```python
from build123d import *

# Parameters (mm, degrees)
F0_W      = 25
F0_H      = 15
F1_DEPTH  = 6
F3_DEPTH  = 10
F5_D      = 5
F6_W      = 10
F6_H      = 15
F7_DEPTH  = 16
F8_DEPTH  = 25.4
F9_DEPTH  = 10
F10_R     = 1.75
F11_DEPTH = 10


with BuildPart() as f1:
    # F0 (on Top) → F1 (new body)
    with BuildSketch(Plane.XY):
        with BuildLine():
            ThreePointArc((-22.1608236432, 15), (-34.6608236432, 27.5), (-47.1608236432, 15))
            Line((-47.1608236432, 15), (-22.1608236432, 15))
        make_face()
        with Locations((-34.6608236432, 7.5)):
            Rectangle(F0_W, F0_H)
        with BuildLine():
            Line((-22.1608236432, 0), (-47.1608236432, 0))
            ThreePointArc((-47.1608236432, 0), (-34.6608236432, -12.5), (-22.1608236432, 0))
        make_face()
    extrude(amount=F1_DEPTH)

    # F2 (on Top) → F3 (join)
    with BuildSketch(Plane.XY):
        with BuildLine():
            Line((-17.1608236432, 0), (-17.1608236432, 15))
            ThreePointArc((-17.1608236432, 15), (-34.6608236432, 32.5), (-52.1608236432, 15))
            Line((-52.1608236432, 15), (-52.1608236432, 0))
            ThreePointArc((-52.1608236432, 0), (-34.6608236432, -17.5), (-17.1608236432, 0))
        make_face()
    extrude(amount=-F3_DEPTH)

    # F5 (through all)
    with Locations(Plane(origin=(-52.1608236432, 0, 0), x_dir=(0, -1, 0), z_dir=(-1, 0, 0))):
        with Locations((-7.5, -5)):
            Hole(F5_D / 2)

    # F6 (on face) → F7 (cut, through all)
    with BuildSketch(Plane(origin=(0, 0, -10), x_dir=(1, 0, 0), z_dir=(0, 0, -1))):
        Polygon((-39.6608236432, 1.5), (-39.6608236432, 0), (-29.6608236432, 0), (-29.6608236432, 1.5), (-34.6608236432, 1.5), align=None)
        with Locations((-34.6608236432, -7.5)):
            Rectangle(F6_W, F6_H)
        Polygon((-29.6608236432, -15), (-39.6608236432, -15), (-39.6608236432, -16.5), (-34.6608236432, -16.5), (-29.6608236432, -16.5), align=None)
    extrude(amount=-F7_DEPTH, mode=Mode.SUBTRACT)

    # F6 (on face) → F8 (cut)
    with BuildSketch(Plane(origin=(0, 0, -10), x_dir=(1, 0, 0), z_dir=(0, 0, -1))):
        with BuildLine():
            ThreePointArc((-30.6608236432, -22.5), (-31.8323965185, -19.6715728753), (-34.6608236432, -18.5))
            ThreePointArc((-34.6608236432, -18.5), (-37.489250768, -25.3284271247), (-30.6608236432, -22.5))
        make_face()
        with BuildLine():
            ThreePointArc((-30.6608236432, 7.5), (-37.489250768, 10.3284271247), (-34.6608236432, 3.5))
            ThreePointArc((-34.6608236432, 3.5), (-31.8323965185, 4.6715728753), (-30.6608236432, 7.5))
        make_face()
    extrude(amount=-F8_DEPTH, mode=Mode.SUBTRACT)

    # F6 (on face) → F9 (join)
    with BuildSketch(Plane(origin=(0, 0, -10), x_dir=(1, 0, 0), z_dir=(0, 0, -1))):
        with BuildLine():
            ThreePointArc((-30.6608236432, -22.5), (-31.8323965185, -19.6715728753), (-34.6608236432, -18.5))
            ThreePointArc((-34.6608236432, -18.5), (-37.489250768, -25.3284271247), (-30.6608236432, -22.5))
        make_face()
        with BuildLine():
            ThreePointArc((-30.6608236432, 7.5), (-37.489250768, 10.3284271247), (-34.6608236432, 3.5))
            ThreePointArc((-34.6608236432, 3.5), (-31.8323965185, 4.6715728753), (-30.6608236432, 7.5))
        make_face()
    extrude(amount=-F9_DEPTH)

    # F10 (on face) → F11 (cut)
    with BuildSketch(Plane.XY):
        with Locations((-34.6608236432, 30)):
            Circle(F10_R)
        with Locations((-34.6608236432, -15)):
            Circle(F10_R)
    extrude(amount=-F11_DEPTH, mode=Mode.SUBTRACT)


solid = f1.part
```
Could you check a few things on this model? Use its own coordinates, in mm. A direction names the side the tool comes from. Round coordinates to 2 decimals unless told otherwise and drop trailing zeros. Write each loop counter-clockwise with the first axis right and the second up, starting at its lowest first coordinate (ties: lowest second). Pieces come first, ordered by that corner, then holes. Notation, with made-up numbers: M 7,35 L 27,35 A35 cw 27,72 Z; hole C 25.25,47.25 d7. An arc over 180 degrees is marked long. Answer in a Markdown table with one row per item. Add a question column.
Q1. Imagine slicing it at C-C (y = 1). Please give me the cut outline in (x, z).
Q2. Imagine slicing it at B-B (y = 9). Please give me the cut outline in (x, z).
Q3. Will these pins go through, and if not, where does the flat tip stop? pin 1 Ø4 at (x, y) = (-35.5, -9) entering from +Z; pin 2 Ø3 at (x, z) = (-28.5, 0) entering from -Y; pin 3 Ø4 at (x, z) = (-22, -6.5) entering from -Y.
Q4. On a 3-axis mill with a long thin cutter (end or side, diameter ignored), from which of +Z, -Z, +X, -X, +Y, -Y can I reach the whole of each face in a straight line? I mean faces 4 (the flat face through (-39.661, 7, -2)), 5 (the flat face through (-22.161, 7, 3)), 6 (the flat face through (-35, -8, 0)), 7 (the cylindrical face through (-34.936, -12.497, 2.958)). Say none if no direction works.
Q5. Imagine slicing it at D-D (z = -1.5). Please give me the cut outline in (x, y).
Q6. Imagine slicing it at A-A (z = -5). Please give me the cut outline in (x, y).
Q7. If I drill on line 1 (X direction, y = 5, z = -4.25); line 2 (X direction, y = 7.5, z = 3); line 3 (Z direction, x = -45.5, y = 27), over which ranges is the centre line in solid material (lowest first)? Write a range as from..to.
Q8. If we mould it in two halves opening along Z, with no side actions, what happens to faces 1 (the cylindrical face through (-34.386, 27.497, 2.958)), 2 (the cylindrical face through (-23.323, 9.885, -4.249)), 3 (the flat face through (-22, 8, 0))? For each: +Z half, -Z half, draft (parallel to the pull), parting line (faces both ways), or undercut.
Values:
| question | item | result |
|---|---|---|
| 1 | outline | M -52.16,-10 L -39.66,-10 L -39.66,6 L -47.16,6 L -47.16,0 L -52.16,0 Z; M -29.66,-10 L -17.16,-10 L -17.16,0 L -22.16,0 L -22.16,6 L -29.66,6 Z |
| 2 | outline | M -52.16,-10 L -39.66,-10 L -39.66,-7 L -52.16,-7 Z; M -52.16,-3 L -39.66,-3 L -39.66,6 L -47.16,6 L -47.16,0 L -52.16,0 Z; M -29.66,-10 L -17.16,-10 L -17.16,-7 L -29.66,-7 Z; M -29.66,-3 L -17.16,-3 L -17.16,0 L -22.16,0 L -22.16,6 L -29.66,6 Z |
| 3 | pin 1 | z = 0 |
| 3 | pin 2 | y = -16.87 |
| 3 | pin 3 | y = -13.88 |
| 4 | face 4 | +Z, -Z |
| 4 | face 5 | +Z, +X, +Y, -Y |
| 4 | face 6 | +Z |
| 4 | face 7 | +Z, -Y |
| 5 | outline | M -52.16,0 A17.5 ccw -17.16,0 L -17.16,15 A17.5 ccw -52.16,15 Z; hole M -39.66,-1.5 L -29.66,-1.5 L -29.66,16.5 L -39.66,16.5 Z; hole C -34.66,-15 d3.5; hole C -34.66,30 d3.5 |
| 6 | outline | M -52.16,0 A17.5 ccw -17.16,0 L -17.16,5 L -29.66,5 L -29.66,-1.5 L -39.66,-1.5 L -39.66,5 L -52.16,5 Z; M -52.16,10 L -39.66,10 L -39.66,16.5 L -29.66,16.5 L -29.66,10 L -17.16,10 L -17.16,15 A17.5 ccw -52.16,15 Z; hole C -34.66,-15 d3.5; hole C -34.66,30 d3.5 |
| 7 | line 1 | -52.16..-39.66, -29.66..-17.16 |
| 7 | line 2 | -47.16..-39.66, -29.66..-22.16 |
| 7 | line 3 | -10..0 |
| 8 | face 1 | draft |
| 8 | face 2 | undercut |
| 8 | face 3 | +Z half |
